Here's how the part is built. I have some questions about the finished solid (model axes, mm). A direction names the side the tool comes from. Coordinates: 2 decimals unless noted, no trailing zeros. Write each loop counter-clockwise with the first axis right and the second up, starting at its lowest first coordinate (ties: lowest second). Pieces come first, ordered by that corner, then holes. Notation, with made-up numbers: (32, -30.5) -> (77, -30.5) arc R17 ccw to (77, 1.5) -> close; hole circle Ø7 at (19, 24). An arc over 180 degrees is marked (long way). Put each result on its own line as item: value. Start each with the question number.
Item 1: For pin 1 (3 mm diameter, centred on y = 3.5, z = -1, fed in from -X); pin 2 (3 mm diameter, centred on y = 3.5, z = -4.5, fed in from +X); pin 3 (3 mm diameter, centred on x = 2.5, z = -1, fed in from +Y), each with a flat end and sliding along its axis, tell me the tip position at first contact or that it passes through.
Item 2: I want a section at D-D, the plane z = 17.5. List the corners of the cut face in (x, y) for me.
Item 3: I want a section at A-A, the plane x = 5.25. List the corners of the cut face in (y, z) for me.
Item 4: On a 3-axis mill with a long thin cutter (end or side, diameter ignored), from which of +Z, -Z, +X, -X, +Y, -Y can I reach the whole of each face in a straight line? I mean faces 4 (the face through (3, 5, -1)), 5 (the face through (3, 0, -4)), 6 (the face through (0, 3, -4)), 7 (the face through (3, 6, -4)). Say none if no direction works.
Item 5: I need wall thicknesses on line 1 (Z direction, x = 5.25, y = 2.75); line 2 (X direction, y = 1, z = 5.5). Which ranges of each line are inside material? Lowest first, please. Write a range as [from, to].
Item 6: If we mould it in two halves opening along Z, with no side actions, what happens to faces 1 (the face through (1, 3, -1)), 2 (the face through (-2, 3, 19)), 3 (the face through (3, 3, 20.5))? For each: released by +Z, released by -Z, zero draft, split by the parting line, or undercut.
Item 7: I want a section at B-B, the plane y = 4.5. List the corners of the cut face in (x, z) for me, then the cut area to 3 significant figures.
from build123d import *

# Parameters (mm, degrees)
SKETCH1_W           = 6
SKETCH1_H           = 6
BOSS_EXTRUDE1_DEPTH = 18
SKETCH2_W           = 10
SKETCH2_H           = 10
BOSS_EXTRUDE2_DEPTH = 2.5
SKETCH5_W           = 4
SKETCH5_H           = 4
BOSS_EXTRUDE4_DEPTH = 2.5
SKETCH6_W           = 6
SKETCH6_H           = 6
BOSS_EXTRUDE5_DEPTH = 2.5


with BuildPart() as part:
    # Sketch1 → Boss-Extrude1 (new body)
    with BuildSketch(Plane.XY):
        with Locations((3, 3)):
            Rectangle(SKETCH1_W, SKETCH1_H)
    extrude(amount=BOSS_EXTRUDE1_DEPTH)

    # Sketch2 → Boss-Extrude2 (add)
    with BuildSketch(Plane.XY.offset(18)):
        with Locations((3, 3)):
            Rectangle(SKETCH2_W, SKETCH2_H)
    extrude(amount=BOSS_EXTRUDE2_DEPTH)

    # Sketch5 → Boss-Extrude4 (add)
    with BuildSketch(Plane(origin=(0, 0, 0), x_dir=(-1, 0, 0), z_dir=(0, 0, -1))):
        with Locations((-3, 3)):
            Rectangle(SKETCH5_W, SKETCH5_H)
    extrude(amount=BOSS_EXTRUDE4_DEPTH)

    # Sketch6 → Boss-Extrude5 (add)
    with BuildSketch(Plane(origin=(0, 0, -2.5), x_dir=(-1, 0, 0), z_dir=(0, 0, -1))):
        with Locations((-3, 3)):
            Rectangle(SKETCH6_W, SKETCH6_H)
    extrude(amount=BOSS_EXTRUDE5_DEPTH)


solid = part.part
Calculated:
1. pin 1: stops at x = 0
1. pin 2: stops at x = 6
1. pin 3: stops at y = 6
2. outline: (0, 0) -> (6, 0) -> (6, 6) -> (0, 6) -> close
3. outline: (-2, 18) -> (0, 18) -> (0, 0) -> (6, 0) -> (6, 18) -> (8, 18) -> (8, 20.5) -> (-2, 20.5) -> close; (0, -5) -> (6, -5) -> (6, -2.5) -> (0, -2.5) -> close
4. face 4: +X, -X, +Y
4. face 5: -Z, +X, -X, -Y
4. face 6: -Z, -X, +Y, -Y
4. face 7: -Z, +X, -X, +Y
5. line 1: z = [-5, -2.5], [0, 20.5]
5. line 2: x = [0, 6]
6. face 1: undercut
6. face 2: zero draft
6. face 3: released by +Z
7. outline: (-2, 18) -> (0, 18) -> (0, 0) -> (1, 0) -> (1, -2.5) -> (0, -2.5) -> (0, -5) -> (6, -5) -> (6, -2.5) -> (5, -2.5) -> (5, 0) -> (6, 0) -> (6, 18) -> (8, 18) -> (8, 20.5) -> (-2, 20.5) -> close
7. area: 158 mm2
